```python
from build123d import *

# Parameters (mm, degrees)
BOX117_W               = 0.8
BOX117_H               = 17
BOX117_DEPTH           = 0.8
BOX118_W               = 0.8
BOX118_H               = 17
BOX118_DEPTH           = 0.8
CUT062_PLACEMENT_ANGLE = 67


with BuildPart() as cubo117:
    # Box117 → Box117 (new body)
    with BuildSketch(Plane.XY):
        with Locations((0.4, 8.5)):
            Rectangle(BOX117_W, BOX117_H)
    extrude(amount=BOX117_DEPTH)


with BuildPart() as obj1:
    # Box118 → Box118 (new body)
    with BuildSketch(Plane(origin=(0.3, 0, 0.3), x_dir=(1, 0, 0), z_dir=(0, 0, 1))):
        with Locations((0.4, 8.5)):
            Rectangle(BOX118_W, BOX118_H)
    extrude(amount=BOX118_DEPTH)

    # Cut062: cut Cubo117
    add(cubo117.part, mode=Mode.SUBTRACT)


with BuildPart() as obj1_1:
    # Cut062 placement: moved
    add(obj1.part.moved(Location((-199.6, 86, -1.47))).rotate(Axis((-199.6, 86, -1.47), (0, 0, 1)), CUT062_PLACEMENT_ANGLE))


solid = obj1_1.part
```
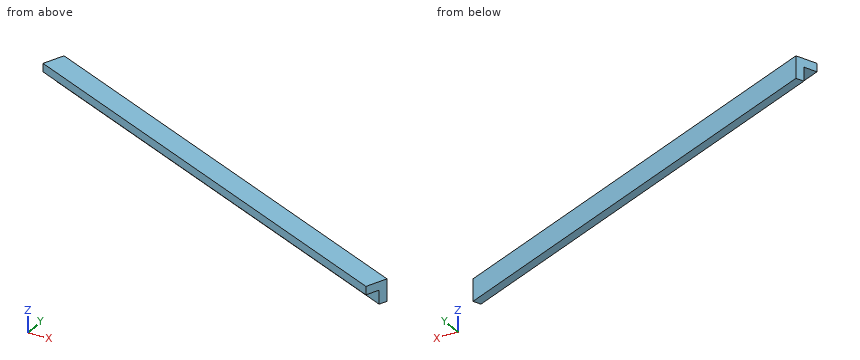
Part model, mm, in its own coordinate system. Round coordinates to 2 decimals unless told otherwise and drop trailing zeros. Loops run counter-clockwise (first coordinate to the right, second up) from the corner with the lowest first, then second, coordinate; pieces in that order, holes last.
Item 1: Cut at A-A, the plane y = 89.5. Give the cut face in (x, z), then the cut area to 3 significant figures.
Item 2: Cut at B-B, the plane z = -1. Give the cut face in (x, y).
Item 3: Cut at C-C, the plane x = -209. Give the cut face in (y, z), then the cut area to 3 significant figures.
Item 4: Drill centre lines: line 1 (X direction, y = 89, z = -0.6); line 2 (Y direction, x = -202, z = -0.8); line 3 (X direction, y = 91.5, z = -0.45). Where is each one in solid material? Low to high.
Item 5: Drop a flat-ended pin along its axis: P1, Ø2, axis at x = -209, y = 88.5, coming from the -Z side. Give the stop position or say it passes through.
A:
1. outline: (-207.08, -0.67) - (-205.8, -0.67) - (-205.8, -1.17) - (-205.03, -1.17) - (-205.03, -0.37) - (-207.08, -0.37) - close
1. area: 0.998 mm2
2. outline: (-214.94, 93.38) - (-199.29, 86.74) - (-199.17, 87.01) - (-214.82, 93.65) - close
3. outline: (90.32, -0.67) - (90.86, -0.67) - (90.86, -1.17) - (91.19, -1.17) - (91.19, -0.37) - (90.32, -0.37) - close
3. area: 0.424 mm2
4. line 1: x = -205.9 to -203.85
4. line 2: y = 87.89 to 88.21
4. line 3: x = -211.79 to -209.74
5. P1: passes through
